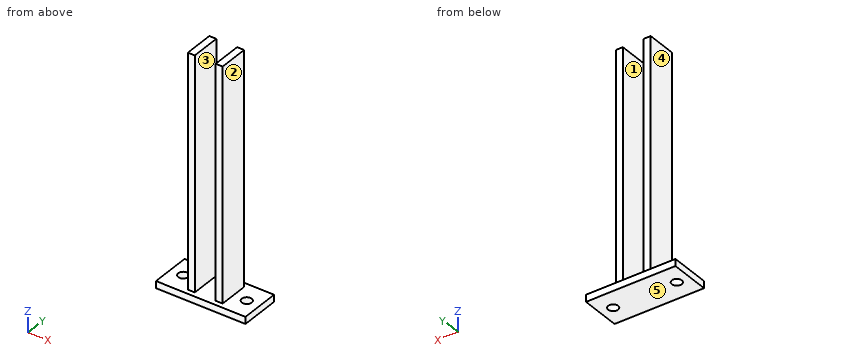
from build123d import *

# Parameters (mm, degrees)
F0_W     = 40
F0_H     = 7
F1_DEPTH = 90
F4_D     = 10
F5_W     = 7
F5_H     = 240
F6_DEPTH = 15
F7_DEPTH = 15


# Not quite as in the source:
# - a feature names something its author has since deleted; it is built from what else it names


with BuildPart() as f1:
    # F0 (on Right) → F1 (new body)
    with BuildSketch(Plane.YZ):
        with Locations((0, 3.5)):
            Rectangle(F0_W, F0_H)
    extrude(amount=F1_DEPTH)

    # F4 (through all)
    with Locations(Plane(origin=(0, 0, 0), x_dir=(1, 0, 0), z_dir=(0, 0, -1))):
        with Locations((13, 0), (77, 0)):
            Hole(F4_D / 2)

    # F5 (on Front) → F6 (join)
    with BuildSketch(Plane.XZ):
        with Locations((60, 120)):
            Rectangle(F5_W, F5_H)
        with Locations((32, 120)):
            Rectangle(F5_W, F5_H)
    extrude(amount=F6_DEPTH)

    # F7 (add): faces of the model
    f7_faces = [f1.faces().sort_by_distance(p)[0] for p in [
        (32, 0, 123.5),
        (60, 0, 123.5),
    ]]
    extrude(f7_faces, amount=F7_DEPTH)


solid = f1.part
For this review, take the finished solid that the model builds, in its own axes (mm). Face numbers are marked on the shaded views. A direction names the side the tool comes from. Round coordinates to 2 decimals unless told otherwise and drop trailing zeros. Loops run counter-clockwise (first coordinate to the right, second up) from the corner with the lowest first, then second, coordinate; pieces in that order, holes last. Notation, with made-up numbers: (60, 2.25) - (103, 2.25) arc R24 ccw to (103, 14.25) - close; hole circle Ø10 at (48.25, 47). An arc over 180 degrees is marked (long way). Use one line per item in the form item = value.
Item 1: Consider section B-B on z = 108. Write out the cut boundary in (x, y), then the cut area to 3 significant figures.
Answers:
outline = (28.5, -15) - (35.5, -15) - (35.5, 15) - (28.5, 15) - close; (56.5, -15) - (63.5, -15) - (63.5, 15) - (56.5, 15) - close
area = 420 mm^2
Item 2: Consider section A-A on x = 13. Write out the cut boundary in (y, z).
Answers:
outline = (-20, 0) - (-5, 0) - (-5, 7) - (-20, 7) - close; (5, 0) - (20, 0) - (20, 7) - (5, 7) - close
Item 3: Clearance check with flat-ended pins moving along their axes: P1, Ø9, axis at y = -1.5, z = 70, coming from the -X side; P2, Ø6, axis at x = 35.5, z = 206.5, coming from the -Y side; P3, Ø1, axis at y = 0, z = 202, coming from the +X side. State where each tip first meets the part, or that it passes through.
Answers:
P1 = 28.5
P2 = -15
P3 = 63.5
Item 4: Consider section D-D on x = 42. Write out the cut boundary in (y, z).
Answers:
outline = (-20, 0) - (20, 0) - (20, 7) - (-20, 7) - close
Item 5: Mouldability with a two-part tool opening along X and no side actions: class the marked faces 3, 4 and 5 as +X half, -X half, draft (parallel to the pull), parting line (faces both ways), or undercut.
Answers:
face_3 = undercut
face_4 = -X half
face_5 = draft
Item 6: Consider section C-C on y = 0. Write out the cut boundary in (x, z).
Answers:
outline = (0, 0) - (8, 0) - (8, 7) - (0, 7) - close; (18, 0) - (72, 0) - (72, 7) - (63.5, 7) - (63.5, 240) - (56.5, 240) - (56.5, 7) - (35.5, 7) - (35.5, 240) - (28.5, 240) - (28.5, 7) - (18, 7) - close; (82, 0) - (90, 0) - (90, 7) - (82, 7) - close
Item 7: For line 1 (X direction, y = -3.5, z = 54.5); line 2 (Y direction, x = 13, z = 2); line 3 (Z direction, x = 43, y = -18), list the stretches that pass through material, from the lowest coordinate up.
Answers:
line_1 = 28.5 to 35.5, 56.5 to 63.5
line_2 = -20 to -5, 5 to 20
line_3 = 0 to 7
Item 8: Tool access review of the marked faces 1 and 2: name each direction out of +Z, -Z, +X, -X, +Y, -Y from which nothing blocks a thin tool from reaching the whole face with its end or side.
Answers:
face_1 = +Z, +Y, -Y
face_2 = +Z, +X, +Y, -Y
